CAD build for the part. Positions are in the model's coordinates, mm. A direction names the side the tool comes from. Round coordinates to 2 decimals unless told otherwise and drop trailing zeros. Write each loop counter-clockwise with the first axis right and the second up, starting at its lowest first coordinate (ties: lowest second). Pieces come first, ordered by that corner, then holes. Notation, with made-up numbers: (62, 25) - (79, 25) arc R12 cw to (79, 46) - close; hole circle Ø10 at (56, -16). An arc over 180 degrees is marked (long way). Put each result on its own line as item: value. Start each with the question number.
Item 1: Cut at D-D (y = 0.9). Give the cut face in (x, z).
Item 2: Cut at A-A (x = 28). Give the cut face in (y, z), and give its area (3 significant figures).
Item 3: 3-axis set-ups, long thin cutter, end or side, ignore diameter. For faces 5 (the flat face through (5, 1, -18)), 6 (the flat face through (-36, 1.5, 30)), 7 (the flat face through (-12, 2, -4)): which of +Z, -Z, +X, -X, +Y, -Y reach the whole face in a straight line?
Item 4: Pin check, flat tips, straight feed: pin 1 Ø3 at (x, z) = (28, -35) entering from +Y; pin 2 Ø1.5 at (x, z) = (27.5, 29) entering from +Y. Stop position of each tip, or through.
Item 5: Cut at B-B (z = -35). Give the cut face in (x, y), and give its area (3 significant figures).
Item 6: Mould opens along X. For faces 1 (the flat face through (20, 1, 3)), 2 (the flat face through (-38.5, 1, -3)), 3 (the flat face through (5, 1, 23)), 4 (the cylindrical face through (30.9, 1.01, 30.93)) say: released by +X, released by -X, zero draft, split by the parting line, or undercut.
Item 7: Cut at C-C (z = -9). Give the cut face in (x, y).
Item 8: Drill centre lines: line 1 (X direction, y = 1, z = -35); line 2 (X direction, y = 1.75, z = 28); line 3 (X direction, y = 0.8, z = -7.5). Where is each one in solid material? Low to high. Write a range as from..to.
```python
from build123d import *

# Parameters (mm, degrees)
SKETCH_1_W          = 70
SKETCH_1_H          = 70
SKETCH_1_R          = 1.7
SKETCH_1_W_2        = 30
SKETCH_1_H_2        = 41
EXTRUDE_1_DEPTH     = 2
FILLET_1_R          = 2
FILLET_2_R          = 1
CUT_EXTRUDE_START   = -0.5
SKETCH_2_R          = 2.5
SKETCH_2_R_2        = 1.7
CUT_EXTRUDE_1_DEPTH = 0.5


with BuildPart() as part:
    # 草图1 → 凸台-拉伸1 (new body)
    with BuildSketch(Plane(origin=(0, 0, 0), x_dir=(1, 0, 0), z_dir=(0, 1, 0))):
        with Locations((-3.5, 3.5)):
            Rectangle(SKETCH_1_W, SKETCH_1_H)
        with Locations(Location((28, -28, 0), (0, 0, 270))):
            Circle(SKETCH_1_R, mode=Mode.SUBTRACT)
        with Locations(Location((28, 35, 0), (0, 0, 270))):
            Circle(SKETCH_1_R, mode=Mode.SUBTRACT)
        with Locations(Location((-35, -28, 0), (0, 0, 90))):
            Circle(SKETCH_1_R, mode=Mode.SUBTRACT)
        with Locations(Location((-35, 35, 0), (0, 0, 90))):
            Circle(SKETCH_1_R, mode=Mode.SUBTRACT)
        with Locations((5, -2.5)):
            Rectangle(SKETCH_1_W_2, SKETCH_1_H_2, mode=Mode.SUBTRACT)
    extrude(amount=EXTRUDE_1_DEPTH)

    # 圆角1
    fillet_1_edges = [part.edges().sort_by_distance(p)[0] for p in [
        (-38.5, 1, -38.5),
        (31.5, 1, -38.5),
        (31.5, 1, 31.5),
        (-38.5, 1, 31.5),
    ]]
    fillet(fillet_1_edges, radius=FILLET_1_R)

    # 圆角2
    fillet_2_edges = [part.edges().sort_by_distance(p)[0] for p in [
        (-10, 1, -18),
        (-10, 1, 23),
        (20, 1, 23),
        (20, 1, -18),
    ]]
    fillet(fillet_2_edges, radius=FILLET_2_R)

    # 草图2 → 切除-拉伸1 (cut)
    # profile 1 of 4: a face of its own
    with BuildSketch(Plane(origin=(0, 2, 0), x_dir=(1, 0, 0), z_dir=(0, 1, 0)).offset(CUT_EXTRUDE_START)):
        with Locations(Location((-35, 35, 0), (0, 0, 270))):
            Circle(SKETCH_2_R)
        with Locations(Location((-35, 35, 0), (0, 0, 90))):
            Circle(SKETCH_2_R_2, mode=Mode.SUBTRACT)
    # profile 2 of 4: a face of its own
    with BuildSketch(Plane(origin=(0, 2, 0), x_dir=(1, 0, 0), z_dir=(0, 1, 0)).offset(CUT_EXTRUDE_START)):
        with Locations(Location((28, 35, 0), (0, 0, 270))):
            Circle(SKETCH_2_R)
        with Locations(Location((28, 35, 0), (0, 0, 270))):
            Circle(SKETCH_2_R_2, mode=Mode.SUBTRACT)
    # profile 3 of 4: a face of its own
    with BuildSketch(Plane(origin=(0, 2, 0), x_dir=(1, 0, 0), z_dir=(0, 1, 0)).offset(CUT_EXTRUDE_START)):
        with Locations(Location((28, -28, 0), (0, 0, 270))):
            Circle(SKETCH_2_R)
        with Locations(Location((28, -28, 0), (0, 0, 270))):
            Circle(SKETCH_2_R_2, mode=Mode.SUBTRACT)
    # profile 4 of 4: a face of its own
    with BuildSketch(Plane(origin=(0, 2, 0), x_dir=(1, 0, 0), z_dir=(0, 1, 0)).offset(CUT_EXTRUDE_START)):
        with Locations(Location((-35, -28, 0), (0, 0, 270))):
            Circle(SKETCH_2_R)
        with Locations(Location((-35, -28, 0), (0, 0, 90))):
            Circle(SKETCH_2_R_2, mode=Mode.SUBTRACT)
    extrude(amount=CUT_EXTRUDE_1_DEPTH, mode=Mode.SUBTRACT)


solid = part.part
```
Output values:
1. outline: (-38.5, -36.5) arc R2 ccw to (-36.5, -38.5) - (29.5, -38.5) arc R2 ccw to (31.5, -36.5) - (31.5, 29.5) arc R2 ccw to (29.5, 31.5) - (-36.5, 31.5) arc R2 ccw to (-38.5, 29.5) - close; hole circle Ø3.4 at (-35, -35); hole circle Ø3.4 at (-35, 28); hole (-10, -17) arc R1 ccw to (-9, -18) - (19, -18) arc R1 ccw to (20, -17) - (20, 22) arc R1 ccw to (19, 23) - (-9, 23) arc R1 ccw to (-10, 22) - close; hole circle Ø3.4 at (28, -35); hole circle Ø3.4 at (28, 28)
2. outline: (0, -38.5) - (2, -38.5) - (2, -37.5) - (1.5, -37.5) - (1.5, -36.7) - (0, -36.7) - close; (0, -33.3) - (1.5, -33.3) - (1.5, -32.5) - (2, -32.5) - (2, 25.5) - (1.5, 25.5) - (1.5, 26.3) - (0, 26.3) - close; (0, 29.7) - (1.5, 29.7) - (1.5, 30.5) - (2, 30.5) - (2, 31.5) - (0, 31.5) - close
2. area: 125 mm2
3. face 5: +Y, -Y
3. face 6: +Y
3. face 7: +Z, -Z, +X, -X, +Y
4. pin 1: through
4. pin 2: y = 1.5
5. outline: (-38.5, 0) - (-36.7, 0) - (-36.7, 1.5) - (-37.5, 1.5) - (-37.5, 2) - (-38.5, 2) - close; (-33.3, 0) - (26.3, 0) - (26.3, 1.5) - (25.5, 1.5) - (25.5, 2) - (-32.5, 2) - (-32.5, 1.5) - (-33.3, 1.5) - close; (29.7, 0) - (31.5, 0) - (31.5, 2) - (30.5, 2) - (30.5, 1.5) - (29.7, 1.5) - close
5. area: 125 mm2
6. face 1: undercut
6. face 2: released by -X
6. face 3: undercut
6. face 4: released by +X
7. outline: (-38.5, 0) - (-10, 0) - (-10, 2) - (-38.5, 2) - close; (20, 0) - (31.5, 0) - (31.5, 2) - (20, 2) - close
8. line 1: -38.5..-36.7, -33.3..26.3, 29.7..31.5
8. line 2: -38.5..-37.5, -32.5..25.5, 30.5..31.5
8. line 3: -38.5..-10, 20..31.5
